Read the model definition and answer for the solid it produces. Units are mm, in the model's axes. A direction names the side the tool comes from. Give positions to 0.01 mm unless a question says otherwise; leave off trailing zeros. Order: outer loops, then holes, each group sorted by start corner. A loop starts at its lowest first (then second) coordinate and runs counter-clockwise, first axis right, second up.
Item 1: The mould has two halves that part along Y. Classify faces 3 (the face through (-0.74, -41.54, 6.37)), 4 (the face through (-3, -50, 1)), 5 (the face through (-1.5, -1, 7)), 6 (the face through (-3, 50, 1)): +Y half, -Y half, draft (parallel to the pull), parting line (faces both ways), or undercut.
Item 2: Which of the six approach directions +Z, -Z, +X, -X, +Y, -Y give full straight-line access (tool end or side, diameter ignored) to faces 1 (the face through (-7, -1, 1.5)), 2 (the face through (-0.74, 44.96, 6.37))?
Item 3: A cutting plane is placed at D-D (x = -4.5). Write down the section's boundary in (y, z), plus the area to 3 significant figures.
Item 4: A cutting plane is placed at B-B (z = 6.75). Write down the section's boundary in (x, y).
Item 5: Given pin 1 Ø1 at (y, z) = (1, 10.5) entering from -X; pin 2 Ø4 at (x, z) = (-4, 10.5) entering from +Y, each flat-ended and moving along its own axis, determine where each tip first touches the part or whether it passes through.
Item 6: A cutting plane is placed at A-A (y = -43.25). Write down the section's boundary in (x, z), plus the area to 3 significant figures.
Item 7: A cutting plane is placed at C-C (y = -9.5). Write down the section's boundary in (x, z).
Item 8: Find the intervals of material crossed by line 1 along Y through (x, z) = (-0.35, 6.75); line 2 along Z through (x, y) = (-0.35, 43.25); line 3 along X through (y, z) = (-15, 9.25), in increasing order.
Autodesk Inventor part; units mm, degrees
ref_plane "YZ Plane" through (0, 0, 0) normal (1, 0, 0) x (0, 1, 0)
ref_plane "XZ Plane" through (0, 0, 0) normal (0, 1, 0) x (-1, 0, 0)
ref_plane "XY Plane" through (0, 0, 0) normal (0, 0, 1) x (1, 0, 0)
sketch "Szkic1" plane through (0, 0, 0) normal (0, 1, 0) x (-1, 0, 0)
  line L0 (0, 0) -> (0, 12)
  line L1 (0, 12) -> (1.5, 12)
  line L2 (1.5, 12) -> (1.5, 1.5)
  line L3 (1.5, 1.5) -> (12, 1.5)
  line L4 (12, 1.5) -> (12, 0)
  line L5 (12, 0) -> (0, 0)
  dimension "d0" = 12
  dimension "d1" = 1.5
  dimension "d2" = 10.5
  dimension "d3" = 10.5
extrude "Wyciągnięcie proste1" add sketch "Szkic1" along normal mid plane 100
sketch "Szkic2" plane through (-1.5, -50, 12) normal (-1, 0, 0) x (0, 0, 1)
  line L0 (0, 100) -> (0, 0)
  line L1 (0, 0) -> (-10.5, 0)
  point P0 (-12, 50)
  point P1 (-5.25, 6.75)
  dimension "d6" = 6.75
  dimension "d7" = 5.25
hole "Otwór1" at (-1.5, -43.25, 6.75) direction (1, 0, 0) diameter 3.5 end through all
mirror "Odbij1" about plane through (0, 0, 0) normal (0, 1, 0) of "Otwór1"
properties part number "bepf_platforma_rama_lacznik_pionowy" material "Aluminium 6061"
Response values:
1. face 3: undercut
1. face 4: -Y half
1. face 5: draft
1. face 6: +Y half
2. face 1: +Z, -X, +Y, -Y
2. face 2: +X, -X
3. outline: (-50, 0) - (50, 0) - (50, 1.5) - (-50, 1.5) - close
3. area: 150 mm2
4. outline: (-1.5, -50) - (0, -50) - (0, -45) - (-1.5, -45) - close; (-1.5, -41.5) - (0, -41.5) - (0, 41.5) - (-1.5, 41.5) - close; (-1.5, 45) - (0, 45) - (0, 50) - (-1.5, 50) - close
5. pin 1: stops at x = -1.5
5. pin 2: passes through
6. outline: (-12, 0) - (0, 0) - (0, 5) - (-1.5, 5) - (-1.5, 1.5) - (-12, 1.5) - close; (-1.5, 8.5) - (0, 8.5) - (0, 12) - (-1.5, 12) - close
6. area: 28.5 mm2
7. outline: (-12, 0) - (0, 0) - (0, 12) - (-1.5, 12) - (-1.5, 1.5) - (-12, 1.5) - close
8. line 1: y = -50 to -45, -41.5 to 41.5, 45 to 50
8. line 2: z = 0 to 5, 8.5 to 12
8. line 3: x = -1.5 to 0
